```python
from build123d import *

# Parameters (mm, degrees)
SKETCH_1_R          = 20
SKETCH_1_R_2        = 1.7
EXTRUDE_1_DEPTH     = 5
SKETCH_2_R          = 1.7
CUT_EXTRUDE_1_DEPTH = 5


with BuildPart() as part:
    # 草图1 → 凸台-拉伸1 (new body)
    with BuildSketch(Plane.XY):
        Circle(SKETCH_1_R)
        with Locations((0, 8)):
            Circle(SKETCH_1_R_2, mode=Mode.SUBTRACT)
        with Locations((8, 0)):
            Circle(SKETCH_1_R_2, mode=Mode.SUBTRACT)
        with Locations((0, -8)):
            Circle(SKETCH_1_R_2, mode=Mode.SUBTRACT)
        with Locations((-8, 0)):
            Circle(SKETCH_1_R_2, mode=Mode.SUBTRACT)
    extrude(amount=EXTRUDE_1_DEPTH)

    # 草图2 → 切除-拉伸1 (cut)
    with BuildSketch(Plane.XY.offset(5)):
        with Locations((0, 14)):
            Circle(SKETCH_2_R)
        with Locations((12.124355653, 7)):
            Circle(SKETCH_2_R)
        with Locations((12.124355653, -7)):
            Circle(SKETCH_2_R)
        with Locations((0, -14)):
            Circle(SKETCH_2_R)
        with Locations((-12.124355653, -7)):
            Circle(SKETCH_2_R)
        with Locations((-12.124355653, 7)):
            Circle(SKETCH_2_R)
    extrude(amount=-CUT_EXTRUDE_1_DEPTH, mode=Mode.SUBTRACT)


solid = part.part
```
Verification items for the finished model (mm, model axes). Give positions to 0.01 mm unless a question says otherwise; leave off trailing zeros. Order: outer loops, then holes, each group sorted by start corner. A loop starts at its lowest first (then second) coordinate and runs counter-clockwise, first axis right, second up. Notation, with made-up numbers: (-10.5, 20) - (44.5, 20) arc R26 ccw to (44.5, 49) - close; hole circle Ø6 at (78.5, 12.5). An arc over 180 degrees is marked (long way). Answer as CSV lines item,"result". Start each with the question number.
Item 1: Mould release check, pull along X, two halves, no side actions. Record for faces 1 (the face through (-4.336, -19.524, 2.465)), 2 (the face through (-9.35, -1.03, 2.46)), 3 (the face through (0, 0, 0)): released by +X, released by -X, zero draft, split by the parting line, or undercut.
Item 2: Section check C-C, the plane x = 7.5. Record the boundary of the cut face in (y, z).
Item 3: Gauge pin test, flat ends, axial feed: pin 1 (3 mm diameter, centred on y = 11, z = 4.5, fed in from +X); pin 2 (2 mm diameter, centred on x = 12.12, y = -7, fed in from +Z); pin 3 (1.5 mm diameter, centred on y = -6.5, z = 4, fed in from +X). Record the tip position at first contact, or that the pin passes through.
Item 4: Section check B-B, the plane z = 4.05. State how many separate pieces and enclosed holes the cut face has, plus the area to 3 significant figures.
Item 5: Section check A-A, the plane y = 0. Record the boundary of the cut face in (x, z).
Item 6: Section check D-D, the plane y = 8. Record the boundary of the cut face in (x, z).
Item 7: Material ranges on L1, parallel to Y at x = 0, z = 2.05; L2, parallel to Y at x = 13.5, z = 2.65; L3, parallel to X at y = -5.5, z = 0.95, recorded low to high.
Filled in:
1,face 1,"split by the parting line"
1,face 2,"undercut"
1,face 3,"zero draft"
2,outline,"(-18.54, 0) - (-1.62, 0) - (-1.62, 5) - (-18.54, 5) - close; (1.62, 0) - (18.54, 0) - (18.54, 5) - (1.62, 5) - close"
3,pin 1,"x = 17.6"
3,pin 2,"through"
3,pin 3,"x = 19.16"
4,separate pieces,"1"
4,enclosed holes,"10"
4,area,"1,170 mm^2"
5,outline,"(-20, 0) - (-9.7, 0) - (-9.7, 5) - (-20, 5) - close; (-6.3, 0) - (6.3, 0) - (6.3, 5) - (-6.3, 5) - close; (9.7, 0) - (20, 0) - (20, 5) - (9.7, 5) - close"
6,outline,"(-18.33, 0) - (-13.5, 0) - (-13.5, 5) - (-18.33, 5) - close; (-10.75, 0) - (-1.7, 0) - (-1.7, 5) - (-10.75, 5) - close; (1.7, 0) - (10.75, 0) - (10.75, 5) - (1.7, 5) - close; (13.5, 0) - (18.33, 0) - (18.33, 5) - (13.5, 5) - close"
7,L1,"-20 to -15.7, -12.3 to -9.7, -6.3 to 6.3, 9.7 to 12.3, 15.7 to 20"
7,L2,"-14.76 to -8, -6 to 6, 8 to 14.76"
7,L3,"-19.23 to -12.92, -11.32 to 11.32, 12.92 to 19.23"
